```python
from build123d import *

# Parameters (mm, degrees)
TORUS_R              = 2.5
TORUS_ROLL_ANGLE     = 90
CYLINDER_R           = 2.5
CYLINDER_DEPTH       = 80
CYLINDER_PITCH_ANGLE = 90


with BuildPart() as torus:
    # Torus → Torus (revolve)
    with BuildSketch(Plane.XZ):
        with Locations((10, 0)):
            Circle(TORUS_R)
    revolve(axis=Axis((0, 0, 0), (0, 0, 1)))


with BuildPart() as torus_1:
    # Torus roll: moved
    add(torus.part.rotate(Axis((0, 0, 0), (1, 0, 0)), TORUS_ROLL_ANGLE))


with BuildPart() as torus_2:
    # Torus placement: moved
    add(torus_1.part)


with BuildPart() as fusion:
    # Cylinder → Cylinder (new body)
    with BuildSketch(Plane.XY):
        Circle(CYLINDER_R)
    extrude(amount=CYLINDER_DEPTH)


with BuildPart() as fusion_1:
    # Cylinder pitch: moved
    add(fusion.part.rotate(Axis((0, 0, 0), (0, 1, 0)), CYLINDER_PITCH_ANGLE))


with BuildPart() as fusion_2:
    # Cylinder placement: moved
    add(fusion_1.part.moved(Location((10, 0, 0))))

    # Fusion: union Torus
    add(torus_2.part)


solid = fusion_2.part
```
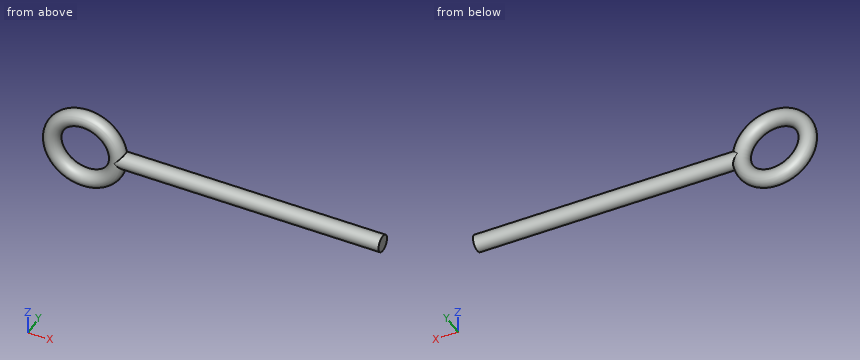
Check sheet for the modelled part. Datum: model origin and axes. Units: mm. Round coordinates to 2 decimals unless told otherwise and drop trailing zeros. Write each loop counter-clockwise with the first axis right and the second up, starting at its lowest first coordinate (ties: lowest second). Pieces come first, ordered by that corner, then holes. Notation, with made-up numbers: (-36.5, -23) -> (-7.5, -23) arc R3 ccw to (-7.5, -19) -> close; hole circle Ø6 at (78, 80.5). An arc over 180 degrees is marked (long way). One line per question, with ' | ' between items. Start each with the question number.
1. Sectioned sample at A-A, the plane z = 0. Record the cut outline in (x, y).
2. Sectioned sample at B-B, the plane y = 0. Record the cut outline in (x, z), then the cut area to 3 significant figures.
3. Sectioned sample at C-C, the plane x = 59.5. Record the cut outline in (y, z), then the cut area to 3 significant figures.
4. Scan lines: line 1 along X through (y, z) = (0.2, 3); line 2 along Z through (x, y) = (-5.5, 2.05); line 3 along X through (y, z) = (-0.5, 3.5). Record each from-to range of solid material in increasing order. Write a range as from..to.
5. Depth check by flat-ended pin: pin 1 (3 mm diameter, centred on y = -2, z = 4, fed in from +X); pin 2 (1 mm diameter, centred on y = -1, z = 4, fed in from -X); pin 3 (1.5 mm diameter, centred on x = 20.5, z = 2, fed in from -Y); pin 4 (4 mm diameter, centred on x = 56, z = -5, fed in from +Y). Enter the tip coordinate at first touch or a pass-through.
Taken from the geometry:
1) outline: circle Ø5 at (-10, 0); (10, -2.5) -> (90, -2.5) -> (90, 2.5) -> (10, 2.5) arc R2.5 ccw to start
2) outline: (12.25, -2.5) -> (90, -2.5) -> (90, 2.5) -> (12.25, 2.5) arc R12.5 ccw (long way) to start; hole circle Ø15 at (0, 0) | area: 702 mm^2
3) outline: circle Ø5 at (0, 0) | area: 19.6 mm^2
4) line 1: x = -12.13..-6.88, 6.88..12.13 | line 2: z = -10.02..-6.57, 6.57..10.02 | line 3: x = -11.95..-6.69, 6.69..11.95
5) pin 1: stops at x = 11.97 | pin 2: stops at x = -11.87 | pin 3: stops at y = -2.17 | pin 4: passes through
